```python
from build123d import *

# Parameters (mm, degrees)
CUT_EXTRUDE1_DEPTH                  = 72.281133549
CUT_EXTRUDE1_DEPTH_BACK             = 72.281133549
SKETCH3_OUTSIDE_W                   = 54.458
SKETCH3_OUTSIDE_H                   = 54.458
SKETCH3_OUTSIDE_W_2                 = 20
SKETCH3_OUTSIDE_H_2                 = 34.409301068
F_8_32_TAPPED_HOLE1_AT_2_COUNT      = 2
F_8_32_TAPPED_HOLE1_AT_2_PITCH      = 43.829214002
F_8_32_TAPPED_HOLE1_AT_3_COUNT      = 2
F_8_32_TAPPED_HOLE1_AT_3_PITCH      = 20
F_8_32_TAPPED_HOLE1_AT_4_COUNT      = 2
F_8_32_TAPPED_HOLE1_AT_4_PITCH      = 39
F_1_8_0_1250_DOWEL_HOLE1_AT_2_COUNT = 2
F_1_8_0_1250_DOWEL_HOLE1_AT_2_PITCH = 39
F_8_32_TAPPED_HOLE2_D               = 3.4544
F_8_32_TAPPED_HOLE2_DEPTH           = 10.71
F_8_32_TAPPED_HOLE2_TIP             = 1.037806461
CUT_EXTRUDE3_DEPTH                  = 50.598387071
CUT_EXTRUDE3_DEPTH_BACK             = 50.598387071


with BuildPart() as part:
    # Sketch2 → Revolve1 (revolve)
    with BuildSketch(Plane.XY, mode=Mode.PRIVATE) as revolve1_sk:
        Polygon((-34, 0), (42, 0), (42, 4), (26, 4), (26, 6.7), (25, 6.7), (25, 17.204650534), (-25, 17.204650534), (-25, 6.7), (-27.5, 6.7), (-27.5, 4), (-34, 4), align=None)
    revolve(revolve1_sk.sketch.rotate(Axis((-34, 0, 0), (1, 0, 0)), 180), axis=Axis((-34, 0, 0), (1, 0, 0)))

    # Sketch3 outside → Cut-Extrude1 (cut, two sides: drawn at the far end of the back side and taken through both)
    with BuildSketch(Plane.ZY.offset(25).offset(-CUT_EXTRUDE1_DEPTH_BACK)):
        Rectangle(SKETCH3_OUTSIDE_W, SKETCH3_OUTSIDE_H)
        Rectangle(SKETCH3_OUTSIDE_W_2, SKETCH3_OUTSIDE_H_2, mode=Mode.SUBTRACT)
    extrude(amount=CUT_EXTRUDE1_DEPTH + CUT_EXTRUDE1_DEPTH_BACK, mode=Mode.SUBTRACT)

    # Sketch5 → #8-32 Tapped Hole1 (revolve, cut)
    with BuildSketch(Plane(origin=(19.5, 10, -10), x_dir=(0, 1, 0), z_dir=(1, 0, 0))):
        Polygon((0, 0), (0, 11.747806461), (1.7272, 10.71), (1.7272, 0), align=None)
    f_8_32_tapped_hole1 = revolve(axis=Axis((19.5, 10, -16.35), (0, 0, 1)), mode=Mode.SUBTRACT)

    # #8-32 Tapped Hole1 at 2: #8-32 Tapped Hole1 ×2
    with Locations(*[Vector(-0.889817462812737, -0.4563166475962754, 0) * (i * F_8_32_TAPPED_HOLE1_AT_2_PITCH) for i in range(1, F_8_32_TAPPED_HOLE1_AT_2_COUNT)]):
        add(f_8_32_tapped_hole1, mode=Mode.SUBTRACT)

    # #8-32 Tapped Hole1 at 3: #8-32 Tapped Hole1 ×2
    with Locations(*[(0, -i * F_8_32_TAPPED_HOLE1_AT_3_PITCH, 0) for i in range(1, F_8_32_TAPPED_HOLE1_AT_3_COUNT)]):
        add(f_8_32_tapped_hole1, mode=Mode.SUBTRACT)

    # #8-32 Tapped Hole1 at 4: #8-32 Tapped Hole1 ×2
    with Locations(*[(-i * F_8_32_TAPPED_HOLE1_AT_4_PITCH, 0, 0) for i in range(1, F_8_32_TAPPED_HOLE1_AT_4_COUNT)]):
        add(f_8_32_tapped_hole1, mode=Mode.SUBTRACT)

    # Sketch7 → 1/8 (0.1250) Dowel Hole1 (revolve, cut)
    with BuildSketch(Plane(origin=(19.5, 0, -10), x_dir=(0, 1, 0), z_dir=(1, 0, 0))):
        Polygon((0, 0), (0, 6.953866233), (1.5875, 6), (1.5875, 0), align=None)
    f_1_8_0_1250_dowel_hole1 = revolve(axis=Axis((19.5, 0, -16.35), (0, 0, 1)), mode=Mode.SUBTRACT)

    # 1/8 (0.1250) Dowel Hole1 at 2: 1/8 (0.1250) Dowel Hole1 ×2
    with Locations(*[(-i * F_1_8_0_1250_DOWEL_HOLE1_AT_2_PITCH, 0, 0) for i in range(1, F_1_8_0_1250_DOWEL_HOLE1_AT_2_COUNT)]):
        add(f_1_8_0_1250_dowel_hole1, mode=Mode.SUBTRACT)

    # Mirror1: #8-32 Tapped Hole1, 1/8 (0.1250) Dowel Hole1 across plane
    add(f_8_32_tapped_hole1.mirror(Plane.XY), mode=Mode.SUBTRACT)
    add(f_1_8_0_1250_dowel_hole1.mirror(Plane.XY), mode=Mode.SUBTRACT)

    # Mirror1 copy 1 sketch → Mirror1 copy 1 (revolve, cut)
    with BuildSketch(Plane(origin=(-19.5, -10, 10), x_dir=(0, 1, 0), z_dir=(1, 0, 0))):
        Polygon((0, 0), (0, -11.747806461), (1.7272, -10.71), (1.7272, 0), align=None)
    revolve(axis=Axis((-19.5, -10, 16.35), (0, 0, 1)), mode=Mode.SUBTRACT)

    # Mirror1 copy 2 sketch → Mirror1 copy 2 (revolve, cut)
    with BuildSketch(Plane(origin=(19.5, -10, 10), x_dir=(0, 1, 0), z_dir=(1, 0, 0))):
        Polygon((0, 0), (0, -11.747806461), (1.7272, -10.71), (1.7272, 0), align=None)
    revolve(axis=Axis((19.5, -10, 16.35), (0, 0, 1)), mode=Mode.SUBTRACT)

    # Mirror1 copy 3 sketch → Mirror1 copy 3 (revolve, cut)
    with BuildSketch(Plane(origin=(-19.5, 10, 10), x_dir=(0, 1, 0), z_dir=(1, 0, 0))):
        Polygon((0, 0), (0, -11.747806461), (1.7272, -10.71), (1.7272, 0), align=None)
    revolve(axis=Axis((-19.5, 10, 16.35), (0, 0, 1)), mode=Mode.SUBTRACT)

    # Mirror1 copy 4 sketch → Mirror1 copy 4 (revolve, cut)
    with BuildSketch(Plane(origin=(-19.5, 0, 10), x_dir=(0, 1, 0), z_dir=(1, 0, 0))):
        Polygon((0, 0), (0, -6.953866233), (1.5875, -6), (1.5875, 0), align=None)
    revolve(axis=Axis((-19.5, 0, 16.35), (0, 0, 1)), mode=Mode.SUBTRACT)

    # #8-32 Tapped Hole2
    with Locations(Plane.ZY.offset(34)):
        with Locations((0, 0)):
            Hole(F_8_32_TAPPED_HOLE2_D / 2, depth=F_8_32_TAPPED_HOLE2_DEPTH)
            with Locations((0, 0, -(F_8_32_TAPPED_HOLE2_DEPTH + F_8_32_TAPPED_HOLE2_TIP / 2))):  # 118° drill point
                Cone(0, F_8_32_TAPPED_HOLE2_D / 2, F_8_32_TAPPED_HOLE2_TIP, mode=Mode.SUBTRACT)

    # Sketch12 → Cut-Extrude3 (cut, two sides: drawn at the far end of the back side and taken through both)
    with BuildSketch(Plane.XY.offset(10).offset(-CUT_EXTRUDE3_DEPTH_BACK)):
        with BuildLine():
            Line((-9.9125, -37.391646785), (9.9125, -37.391646785))
            ThreePointArc((9.9125, -37.391646785), (14.862247468, -35.341394253), (16.9125, -30.391646785))
            Line((16.9125, -30.391646785), (16.9125, 2))
            ThreePointArc((16.9125, 2), (14.862247468, 6.949747468), (9.9125, 9))
            Line((9.9125, 9), (-9.9125, 9))
            ThreePointArc((-9.9125, 9), (-14.862247468, 6.949747468), (-16.9125, 2))
            Line((-16.9125, 2), (-16.9125, -30.391646785))
            ThreePointArc((-16.9125, -30.391646785), (-14.862247468, -35.341394253), (-9.9125, -37.391646785))
        make_face()
    extrude(amount=CUT_EXTRUDE3_DEPTH + CUT_EXTRUDE3_DEPTH_BACK, mode=Mode.SUBTRACT)


solid = part.part
```
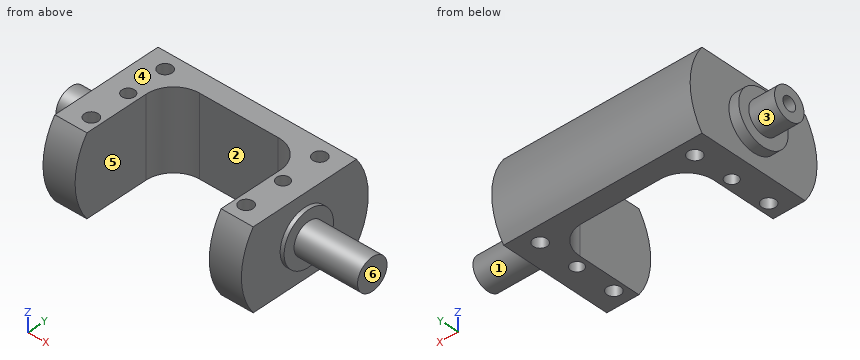
Input: part model. Units: mm. Frame: model coordinates. Face numbers are marked on the shaded views. A direction names the side the tool comes from. Round coordinates to 2 decimals unless told otherwise and drop trailing zeros. Order: outer loops, then holes, each group sorted by start corner. A loop starts at its lowest first (then second) coordinate and runs counter-clockwise, first axis right, second up. Notation, with made-up numbers: (-26.75, 17) - (23.25, 17) arc R15 ccw to (23.25, 31) - close; hole circle Ø2 at (-22.75, 22.25). An arc over 180 degrees is marked (long way). One line per question, with ' | ' between items. Start each with the question number.
1) Ray query, probe 1 along X at (y, z) = (-10, -6.25); probe 2 along X at (y, z) = (10, -3); probe 3 along X at (y, z) = (0, 5.5). Return the intervals inside material, ascending.
2) Set-up query: the marked faces 1, 2 and 3. Return all of +Z, -Z, +X, -X, +Y, -Y with unobstructed straight access to the full face (end or side cutting, diameter ignored); none if empty.
3) Contact query for flat-ended pins moving along their axis: P1, Ø2.5, axis at x = -19.5, y = 0, coming from the -Z side; P2, Ø3, axis at x = 14, z = -6.5, coming from the +Y side; P3, Ø2, axis at x = -19.5, y = 10, coming from the +Z side; P4, Ø12, axis at x = -19, z = -6.5, coming from the -Y side. Output: stop coordinate, or through.
4) Cut plane D-D, the plane z = 5.5. Return the cut outline in (x, y) (1 decimal), then the cut area to 3 significant figures.
5) Cut plane B-B, the plane z = -8.75. Return the cut outline in (x, y) (1 decimal), then the cut area to 3 significant figures.
6) Pull-direction query (X, two-part tool) for the marked faces 4, 5 and 6; classes: +X half, -X half, draft (parallel to the pull), parting line (faces both ways), or undercut.
7) Cut plane C-C, the plane x = -8. Return the cut outline in (y, z).
8) Cut plane A-A, the plane y = 10. Return the cut outline in (x, z), then the cut area to 3 significant figures.
Worked out:
1) probe 1: x = -25 to -21.23, -17.77 to -16.91, 16.91 to 17.77, 21.23 to 25 | probe 2: x = -25 to -21.23, -17.77 to 17.77, 21.23 to 25 | probe 3: x = -27.5 to -21.09, -17.91 to -16.91, 16.91 to 17.91, 21.09 to 26
2) face 1: +X | face 2: +Z, -Z, -Y | face 3: -X
3) P1: stops at z = -3.8 | P2: stops at y = 16.46 | P3: passes through | P4: stops at y = -17.2
4) outline: (-27.5, -3.8) - (-25, -3.8) - (-25, -16.3) - (-16.9, -16.3) - (-16.9, 2) arc R7 cw to (-9.9, 9) - (9.9, 9) arc R7 cw to (16.9, 2) - (16.9, -16.3) - (25, -16.3) - (25, -3.8) - (26, -3.8) - (26, 3.8) - (25, 3.8) - (25, 16.3) - (-25, 16.3) - (-25, 3.8) - (-27.5, 3.8) - close; hole circle Ø3.5 at (-19.5, -10); hole circle Ø3.5 at (-19.5, 10); hole circle Ø3.2 at (-19.5, 0); hole circle Ø3.5 at (19.5, -10); hole circle Ø3.5 at (19.5, 10); hole circle Ø3.2 at (19.5, 0) | area: 769 mm^2
5) outline: (-25, -14.8) - (-16.9, -14.8) - (-16.9, 2) arc R7 cw to (-9.9, 9) - (9.9, 9) arc R7 cw to (16.9, 2) - (16.9, -14.8) - (25, -14.8) - (25, 14.8) - (-25, 14.8) - close; hole circle Ø3.5 at (-19.5, -10); hole circle Ø3.5 at (-19.5, 10); hole circle Ø3.2 at (-19.5, 0); hole circle Ø3.5 at (19.5, -10); hole circle Ø3.5 at (19.5, 10); hole circle Ø3.2 at (19.5, 0) | area: 644 mm^2
6) face 4: draft | face 5: undercut | face 6: +X half
7) outline: (9, -10) - (14, -10) arc R17.2 ccw to (14, 10) - (9, 10) - close
8) outline: (-25, -10) - (-21.23, -10) - (-21.23, 10) - (-25, 10) - close; (-17.77, -10) - (17.77, -10) - (17.77, 10) - (-17.77, 10) - close; (21.23, -10) - (25, -10) - (25, 10) - (21.23, 10) - close | area: 862 mm^2
